from build123d import *

# Parameters (mm, degrees)
F3_D     = 3
F3_DEPTH = 1
F3_TIP   = 0.9012909285
F5_DEPTH = 1.1


with BuildPart() as f1:
    # F0 (on Front) → F1 (revolve)
    with BuildSketch(Plane.XZ):
        Polygon((1.5, 6), (0, 6), (0, 0), (2.753497507, 0), (2.753497507, 0.685), (1.5, 1.82), align=None)
    revolve(axis=Axis((0, 0, 3), (0, 0, -1)))

    # F3
    with Locations(Plane(origin=(0, 0, 0), x_dir=(1, 0, 0), z_dir=(0, 0, -1))):
        with Locations((0, 0)):
            Hole(F3_D / 2, depth=F3_DEPTH)
            with Locations((0, 0, -(F3_DEPTH + F3_TIP / 2))):  # 118° drill point
                Cone(0, F3_D / 2, F3_TIP, mode=Mode.SUBTRACT)

    # F4 (on face) → F5 (cut)
    with BuildSketch(Plane(origin=(0, 0, 0), x_dir=(1, 0, 0), z_dir=(0, 0, -1))):
        with BuildLine():
            ThreePointArc((1.4420504443, -0.4129049722), (1.4854419656, -0.2084758182), (1.5, 0))
            ThreePointArc((1.5, 0), (1.3906683924, 0.5621756153), (1.0786114367, 1.0423998122))
            ThreePointArc((1.0786114367, 1.0423998122), (0.4129049995, 1.4420504365), (-0.3634389987, 1.4553048114))
            ThreePointArc((-0.3634389987, 1.4553048114), (-1.0423998218, 1.0786114275), (-1.4420504443, 0.4129049722))
            ThreePointArc((-1.4420504443, 0.4129049722), (-1.4553048039, -0.363439029), (-1.0786114144, -1.0423998354))
            ThreePointArc((-1.0786114144, -1.0423998354), (-0.412904984, -1.4420504409), (0.3634389987, -1.4553048114))
            ThreePointArc((0.3634389987, -1.4553048114), (1.0423998218, -1.0786114275), (1.4420504443, -0.4129049722))
        make_face()
        with BuildLine():
            ThreePointArc((1.0786114367, 1.0423998122), (1.3906683924, 0.5621756153), (1.5, 0))
            ThreePointArc((1.5, 0), (1.4854419656, -0.2084758182), (1.4420504443, -0.4129049722))
            Line((1.4420504443, -0.4129049722), (1.680441244, 0.4196632286))
            Line((1.680441244, 0.4196632286), (1.0786114367, 1.0423998122))
        make_face()
        with BuildLine():
            ThreePointArc((-0.3634389987, 1.4553048114), (0.4129049995, 1.4420504365), (1.0786114367, 1.0423998122))
            Line((1.0786114367, 1.0423998122), (0.476781605, 1.6651364212))
            Line((0.476781605, 1.6651364212), (-0.3634389987, 1.4553048114))
        make_face()
        with BuildLine():
            Line((1.203659639, -1.2454731926), (1.4420504443, -0.4129049722))
            ThreePointArc((1.4420504443, -0.4129049722), (1.0423998218, -1.0786114275), (0.3634389987, -1.4553048114))
            Line((0.3634389987, -1.4553048114), (1.203659639, -1.2454731926))
        make_face()
        with BuildLine():
            ThreePointArc((-1.4420504443, 0.4129049722), (-1.0423998218, 1.0786114275), (-0.3634389987, 1.4553048114))
            Line((-0.3634389987, 1.4553048114), (-1.203659639, 1.2454731926))
            Line((-1.203659639, 1.2454731926), (-1.4420504443, 0.4129049722))
        make_face()
        with BuildLine():
            Line((-0.476781605, -1.6651364212), (0.3634389987, -1.4553048114))
            ThreePointArc((0.3634389987, -1.4553048114), (-0.412904984, -1.4420504409), (-1.0786114144, -1.0423998354))
            Line((-1.0786114144, -1.0423998354), (-0.476781605, -1.6651364212))
        make_face()
        with BuildLine():
            ThreePointArc((-1.0786114144, -1.0423998354), (-1.4553048039, -0.363439029), (-1.4420504443, 0.4129049722))
            Line((-1.4420504443, 0.4129049722), (-1.680441244, -0.4196632286))
            Line((-1.680441244, -0.4196632286), (-1.0786114144, -1.0423998354))
        make_face()
    extrude(amount=-F5_DEPTH, mode=Mode.SUBTRACT)


solid = f1.part
Work out the finished part from the listing and answer in its coordinate system (mm). A direction names the side the tool comes from. Coordinates: 2 decimals unless noted, no trailing zeros. Write each loop counter-clockwise with the first axis right and the second up, starting at its lowest first coordinate (ties: lowest second). Pieces come first, ordered by that corner, then holes. Notation, with made-up numbers: M 86.25,77 L 123.25,77 A19 ccw 123.25,96 Z; hole C -38.75,68.25 d10. An arc over 180 degrees is marked long. Use one line per item in the form item = value. Start each with the question number.
1. The part is cut by section A-A (z = 0.4). Give the vertices of the cut face in (x, y), plus the area to 3 significant figures.
2. The part is cut by section B-B (z = 5.55). Give the vertices of the cut face in (x, y), plus the area to 3 significant figures.
3. The mould has two halves that part along Y. Classify faces 1 (the face through (-0.05, 0.23, 1.76)), 2 (the face through (-1.2, 1.2, 0)), 3 (the face through (-0.36, -2.73, 0.35)): released by +Y, released by -Y, zero draft, split by the parting line, or undercut.
4. A tool of negligible diameter and unlimited length cuts with its end or side. For faces 4 (the face through (0, 0, 6)), 5 (the face through (-1.5, -0.07, 3.94)), from which of +Z, -Z, +X, -X, +Y, -Y can it reach the whole face along a straight path? Write none if from no direction.
5. Straight lines are drawn through the part: probe 1 along Y at (x, z) = (0.05, 2.3); probe 2 along X at (y, z) = (0.85, 1.2); probe 3 along Z at (x, y) = (-0.1, 1.4). For each, find the intervals that lie inside material, in ascending order. Write a range as from..to.
6. Each of these flat-tipped pins is pushed along its axis until it touches: P1, Ø1.5, axis at y = 1, z = 4, coming from the +X side; P2, Ø1.5, axis at x = 1, z = 4.5, coming from the -Y side. Where does it stop, or does it pass through?
Evaluation:
q1.outline = C 0,0 d5.51; hole M -1.68,0.42 L -1.2,-1.25 L 0.48,-1.67 L 1.68,-0.42 L 1.2,1.25 L -0.48,1.67 Z
q1.area = 16.0 mm^2
q2.outline = C 0,0 d3
q2.area = 7.07 mm^2
q3.face_1 = undercut
q3.face_2 = zero draft
q3.face_3 = split by the parting line
q4.face_4 = +Z, +X, -X, +Y, -Y
q4.face_5 = +Z
q5.probe_1 = -1.5..1.5
q5.probe_2 = -2.01..-0.8, 0.8..2.01
q5.probe_3 = 1.1..6
q6.P1 = 1.48
q6.P2 = -1.48
